from build123d import *

# Parameters (mm, degrees)
SKETCH_1_W        = 9.6
SKETCH_1_H        = 5.6
SKETCH_1_W_2      = 8
SKETCH_1_H_2      = 4
EXTRUDE_1_DEPTH   = 5
EXTRUDE_1_2_DEPTH = 5
EXTRUDE_1_3_DEPTH = 3
SKETCH_3_W        = 8
SKETCH_3_H        = 4
EXTRUDE_2_DEPTH   = 1
FILLET_1_R        = 2
FILLET_2_R        = 0.4


with BuildPart() as part:
    # Эскиз1 → Extrude 1 (new body)
    with BuildSketch(Plane(origin=(0, 0, 0), x_dir=(1, 0, 0), z_dir=(0, 1, 0))):
        with Locations((0.747071049, 17.586951222)):
            Rectangle(SKETCH_1_W, SKETCH_1_H)
        with Locations((0.747071049, 17.586951222)):
            Rectangle(SKETCH_1_W_2, SKETCH_1_H_2, mode=Mode.SUBTRACT)
    extrude(amount=EXTRUDE_1_DEPTH)



with BuildPart() as body_2:
    # Эскиз1 → Extrude 1 2 (new body)
    with BuildSketch(Plane(origin=(0, 0, 0), x_dir=(1, 0, 0), z_dir=(0, 1, 0))):
        with Locations((0.747071049, -15.413048778)):
            Rectangle(SKETCH_1_W, SKETCH_1_H)
        with Locations((0.747071049, -15.413048778)):
            Rectangle(SKETCH_1_W_2, SKETCH_1_H_2, mode=Mode.SUBTRACT)
    extrude(amount=EXTRUDE_1_2_DEPTH)


with BuildPart() as part_1:
    add(part.part)

    add(body_2.part)  # Extrude 1 3 merges body 2
    # Эскиз2 → Extrude 1 3 (add)
    with BuildSketch(Plane(origin=(0, 5, 0), x_dir=(1, 0, 0), z_dir=(0, 1, 0))):
        Polygon((-4.052928951, 20.386951222), (-13.052928951, 20.386951222), (-13.052928951, -18.213048778), (-4.052928951, -18.213048778), (-4.052928951, -12.613048778), (-8.052928951, -12.613048778), (-8.052928951, 14.786951222), (-4.052928951, 14.786951222), align=None)
    extrude(amount=-EXTRUDE_1_3_DEPTH)

    # Эскиз3 → Бобышка-Вытянуть2 (add)
    with BuildSketch(Plane(origin=(0, 5, 0), x_dir=(1, 0, 0), z_dir=(0, 1, 0))):
        with Locations((0.747071049, 17.586951222)):
            Rectangle(SKETCH_3_W, SKETCH_3_H)
        with Locations((0.747071049, -15.413048778)):
            Rectangle(SKETCH_3_W, SKETCH_3_H)
    extrude(amount=-EXTRUDE_2_DEPTH)

    # Скругление1
    fillet_1_edges = [part_1.edges().sort_by_distance(p)[0] for p in [
        (-4.052928951, 2, -17.586951222),
        (-4.052928951, 2, 15.413048778),
        (-8.052928951, 3.5, 12.613048778),
        (-8.052928951, 3.5, -14.786951222),
        (-13.052928951, 3.5, -20.386951222),
        (-13.052928951, 3.5, 18.213048778),
    ]]
    fillet(fillet_1_edges, radius=FILLET_1_R - 0.0001)  # a hair under: the kernel refuses the full size

    # Скругление2
    fillet_2_edges = [part_1.edges().sort_by_distance(p)[0] for p in [
        (5.547071049, 2.5, 18.213048778),
        (5.547071049, 2.5, 12.613048778),
        (5.547071049, 2.5, -14.786951222),
        (5.547071049, 2.5, -20.386951222),
    ]]
    fillet(fillet_2_edges, radius=FILLET_2_R)


solid = part_1.part
Build history of the part. All positions in model axes, mm. A direction names the side the tool comes from. Give positions to 0.01 mm unless a question says otherwise; leave off trailing zeros. Loops run counter-clockwise (first coordinate to the right, second up) from the corner with the lowest first, then second, coordinate; pieces in that order, holes last. Notation, with made-up numbers: (40.5, 19) - (56.5, 19) arc R23 ccw to (56.5, 55) - close; hole circle Ø7 at (29, -26.5). An arc over 180 degrees is marked (long way). Write item = value, one per line. Start each with the question number.
1) Tool access for faces 1 (the flat face through (-10, 2, -1)), 2 (the flat face through (5.547, 2, 15)), 3 (the flat face through (1, 2, -15.587)), 4 (the flat face through (0, 3, 12.613)): list every direction of +Z, -Z, +X, -X, +Y, -Y with a clear straight run to the whole face (end or side of a thin tool).
2) Drop flat-ended pins along their axis: pin 1 Ø0.9 at (y, z) = (3.5, -7) entering from +X; pin 2 Ø2 at (x, z) = (2.5, -18.5) entering from -Y; pin 3 Ø3.5 at (x, z) = (-10.5, 3) entering from -Y; pin 4 Ø1.5 at (x, z) = (-3, -14.5) entering from -Y. Give the stop position or say it passes through.
3) Pull direction X, two halves, no side cores. Call faces 5 (the flat face through (1, 2, 13.413)), 6 (the flat face through (-1, 3, -14.787)), 7 (the cylindrical face through (-7.48, 3.48, -14.19)): +X half, -X half, draft (parallel to the pull), parting line (faces both ways), or undercut.
4) Probe probe 1 along Z at (x, y) = (3.5, 1.55); probe 2 along Z at (x, y) = (-4.75, 4.1); probe 3 along X at (y, z) = (3.95, -4). List the from-to ranges inside material, lowest first. Write a range as from..to.
5) Band-saw the part on C-C on y = 4.4. Give the cut face in (x, z), plus the area to 3 significant figures.
6) Band-saw the part on B-B on x = 1.25. Give the cut face in (y, z).
7) Band-saw the part on D-D on x = -5.5. Give the cut face in (y, z).
8) Band-saw the part on A-A on y = 0.85. Give the cut face in (x, z), plus the area to 3 significant figures.
Final values:
q1.face_1 = +Z, -Z, -X, -Y
q1.face_2 = +Z, -Z, +X, +Y, -Y
q1.face_3 = -Y
q1.face_4 = +X, +Y, -Y
q2.pin_1 = -8.05
q2.pin_2 = 4
q2.pin_3 = 2
q2.pin_4 = 0
q3.face_5 = undercut
q3.face_6 = draft
q3.face_7 = +X half
q4.probe_1 = -20.39..-19.59, -15.59..-14.79, 12.61..13.41, 17.41..18.21
q4.probe_2 = -20.39..-14.79, 12.61..18.21
q4.probe_3 = -13.05..-8.05
q5.outline = (-13.05, -18.39) arc R2 ccw to (-11.05, -20.39) - (5.15, -20.39) arc R0.4 ccw to (5.55, -19.99) - (5.55, -15.19) arc R0.4 ccw to (5.15, -14.79) - (-6.05, -14.79) arc R2 cw to (-8.05, -12.79) - (-8.05, 10.61) arc R2 cw to (-6.05, 12.61) - (5.15, 12.61) arc R0.4 ccw to (5.55, 13.01) - (5.55, 17.81) arc R0.4 ccw to (5.15, 18.21) - (-11.05, 18.21) arc R2 ccw to (-13.05, 16.21) - close
q5.area = 345 mm²
q6.outline = (0, -20.39) - (5, -20.39) - (5, -14.79) - (0, -14.79) - (0, -15.59) - (4, -15.59) - (4, -19.59) - (0, -19.59) - close; (0, 12.61) - (5, 12.61) - (5, 18.21) - (0, 18.21) - (0, 17.41) - (4, 17.41) - (4, 13.41) - (0, 13.41) - close
q7.outline = (1.92, -20.39) - (5, -20.39) - (5, -14.79) - (1.92, -14.79) - close; (1.92, 12.61) - (5, 12.61) - (5, 18.21) - (1.92, 18.21) - close
q8.outline = (-4.24, -20.39) - (5.15, -20.39) arc R0.4 ccw to (5.55, -19.99) - (5.55, -15.19) arc R0.4 ccw to (5.15, -14.79) - (-4.24, -14.79) - close; (-4.24, 12.61) - (5.15, 12.61) arc R0.4 ccw to (5.55, 13.01) - (5.55, 17.81) arc R0.4 ccw to (5.15, 18.21) - (-4.24, 18.21) - close; hole (-3.25, -19.59) - (4.75, -19.59) - (4.75, -15.59) - (-3.25, -15.59) - close; hole (-3.25, 13.41) - (4.75, 13.41) - (4.75, 17.41) - (-3.25, 17.41) - close
q8.area = 45.5 mm²
